Design review of the part built by this model. Coordinates are the model's own, in mm. Face numbers are marked on the shaded views. A direction names the side the tool comes from. Round coordinates to 2 decimals unless told otherwise and drop trailing zeros. Order: outer loops, then holes, each group sorted by start corner. A loop starts at its lowest first (then second) coordinate and runs counter-clockwise, first axis right, second up.
from build123d import *

# Parameters (mm, degrees)
F1_DEPTH = 8.89
F2_R     = 1.1303
F3_DEPTH = 25.4
F4_R     = 1.27
F5_SIZE  = 0.508


with BuildPart() as f1:
    # F0 (on Front) → F1 (new body)
    with BuildSketch(Plane.XZ):
        Polygon((-6.604, 2.286), (6.604, 2.286), (6.604, -2.286), (12.7, -2.286), (12.7, 4.826), (-12.7, 4.826), (-12.7, -2.286), (-6.604, -2.286), align=None)
    extrude(amount=F1_DEPTH)

    # F2 (on face) → F3 (cut)
    with BuildSketch(Plane(origin=(0, 0, -2.286), x_dir=(1, 0, 0), z_dir=(0, 0, -1))):
        with Locations((-9.652, 4.445)):
            Circle(F2_R)
        with Locations((9.652, 4.445)):
            Circle(F2_R)
    extrude(amount=-F3_DEPTH, mode=Mode.SUBTRACT)

    # F4
    f4_edges = [f1.edges().sort_by_distance(p)[0] for p in [
        (-6.604, -4.445, 2.286),
        (6.604, -4.445, 2.286),
        (-12.7, 0, 1.27),
        (-12.7, -8.89, 1.27),
        (12.7, -8.89, 1.27),
        (12.7, 0, 1.27),
    ]]
    fillet(f4_edges, radius=F4_R)

    # F5
    f5_edges = [f1.edges().sort_by_distance(p)[0] for p in [
        (12.7, -4.445, 4.826),
        (12.328026, -0.371974, 4.826),
        (12.328026, -8.518026, 4.826),
        (0, 0, 4.826),
        (0, -8.89, 4.826),
        (-12.328026, -0.371974, 4.826),
        (-12.328026, -8.518026, 4.826),
        (-12.7, -4.445, 4.826),
        (8.5217, -4.445, 4.826),
        (-10.7823, -4.445, 4.826),
    ]]
    chamfer(f5_edges, length=F5_SIZE)


solid = f1.part
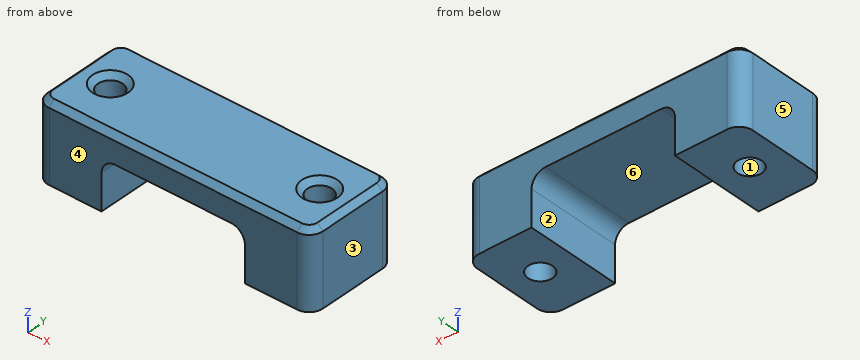
1) Take a section at B-B on x = 0.25. Give the boundary of the cut face in (y, z), plus the area to 3 significant figures.
Results:
outline: (-8.89, 2.29) - (0, 2.29) - (0, 4.32) - (-0.51, 4.83) - (-8.38, 4.83) - (-8.89, 4.32) - close
area: 22.3 mm2
2) To check wall thickness, follow line 1 along X through (y, z) = (-4.5, -1); line 2 along X through (y, z) = (-2.5, -1); line 3 along X through (y, z) = (-4.25, 2.75). State the ranges of each line that lie inside material, in increasing order.
Results:
line 1: x = -12.7 to -10.78, -8.52 to -6.6, 6.6 to 8.52, 10.78 to 12.7
line 2: x = -12.7 to -6.6, 6.6 to 12.7
line 3: x = -12.7 to -10.77, -8.54 to 8.54, 10.77 to 12.7
3) For the marked faces 1 and 2, list the 3-axis set-ups (+Z, -Z, +X, -X, +Y, -Y) from which the entire face can be reached by the end or side of a thin tool; tool diameter is ignored.
Results:
face 1: +Z, -Z
face 2: -Z, +Y, -Y
4) Take a section at D-D on z = 3. Give the boundary of the cut face in (x, y) (3 decimals), plus the area to 3 significant figures.
Results:
outline: (-12.7, -7.62) arc R1.27 ccw to (-11.43, -8.89) - (11.43, -8.89) arc R1.27 ccw to (12.7, -7.62) - (12.7, -1.27) arc R1.27 ccw to (11.43, 0) - (-11.43, 0) arc R1.27 ccw to (-12.7, -1.27) - close; hole circle Ø2.261 at (-9.652, -4.445); hole circle Ø2.261 at (9.652, -4.445)
area: 216 mm2
5) The part is to be moulded in two halves that separate along X. For the marked faces 3, 4, 5 and 6, say which applies: released by +X, released by -X, zero draft, split by the parting line, or undercut.
Results:
face 3: released by +X
face 4: zero draft
face 5: released by -X
face 6: undercut
6) Take a section at C-C on z = -1. Give the boundary of the cut face in (x, y) (3 decimals).
Results:
outline: (-12.7, -7.62) arc R1.27 ccw to (-11.43, -8.89) - (-6.604, -8.89) - (-6.604, 0) - (-11.43, 0) arc R1.27 ccw to (-12.7, -1.27) - close; (6.604, -8.89) - (11.43, -8.89) arc R1.27 ccw to (12.7, -7.62) - (12.7, -1.27) arc R1.27 ccw to (11.43, 0) - (6.604, 0) - close; hole circle Ø2.261 at (-9.652, -4.445); hole circle Ø2.261 at (9.652, -4.445)
7) Take a section at A-A on z = 1.5. Give the boundary of the cut face in (x, y) (3 decimals).
Results:
outline: (-12.7, -7.62) arc R1.27 ccw to (-11.43, -8.89) - (-6.508, -8.89) - (-6.508, 0) - (-11.43, 0) arc R1.27 ccw to (-12.7, -1.27) - close; (6.508, -8.89) - (11.43, -8.89) arc R1.27 ccw to (12.7, -7.62) - (12.7, -1.27) arc R1.27 ccw to (11.43, 0) - (6.508, 0) - close; hole circle Ø2.261 at (-9.652, -4.445); hole circle Ø2.261 at (9.652, -4.445)
8) Clearance check with flat-ended pins moving along their axes: P1, Ø1.5, axis at x = 1, y = -5, coming from the -Z side; P2, Ø3, axis at x = -9.652, y = -4.445, coming from the +Z side. State where each tip first meets the part, or that it passes through.
Results:
P1: stops at z = 2.29
P2: stops at z = 4.69
